Job drawing, mm, ordinate dimensions from the low corner. One solid piece. A direction names the side the tool comes from. Give positions to 0.01 mm unless a question says otherwise; leave off trailing zeros. Order: outer loops, then holes, each group sorted by start corner. A loop starts at its lowest first (then second) coordinate and runs counter-clockwise, first axis right, second up. Notation, with made-up numbers: M 59.5,48 L 78.5,48 A17 cw 78.5,52 Z; hole C -37.75,0 d5. An arc over 180 degrees is marked long. Use CSV: the item, a comma, the result in double quotes. Start each with the question number.
Item 1: Band-saw the part on D-D on y = 2. Write the cut outline in (x, z).
Item 2: Band-saw the part on B-B on z = 5. Write the cut outline in (x, y), plus the area to 3 significant figures.
Item 3: Which spindle directions (+Z, -Z, +X, -X, +Y, -Y) get a long thin tool onto all of the face, cutting with end or side? Do the marked faces 4, 5 and 6. Say none if no direction does.
Item 4: Wall check: line 1 along X through (y, z) = (17.6, 25) (1 decimal); line 2 along Y through (x, z) = (17.5, 43); line 3 along Z through (x, y) = (14.5, 15.75) (1 decimal). Give the ranges that are in metal, low to high.
Item 5: Two-plate mould, pull along X, no slides. Class the marked faces 1, 2 and 3: pulls with the +X half, pulls with the -X half, needs draft (parallel to the pull), parting line crosses it, or undercut.
Item 6: Pin check, flat tips, straight feed: P1, Ø6, axis at x = 33, y = 9.5, coming from the +Z side; P2, Ø3.5, axis at x = 24, y = 12.5, coming from the -Z side; P3, Ø3.5, axis at x = 5, z = 25, coming from the +Y side. Stop position of each tip, or through.
Item 7: Band-saw the part on A-A on x = 5. Write the cut outline in (y, z).
Item 8: Band-saw the part on C-C on x = 25. Write the cut outline in (y, z).
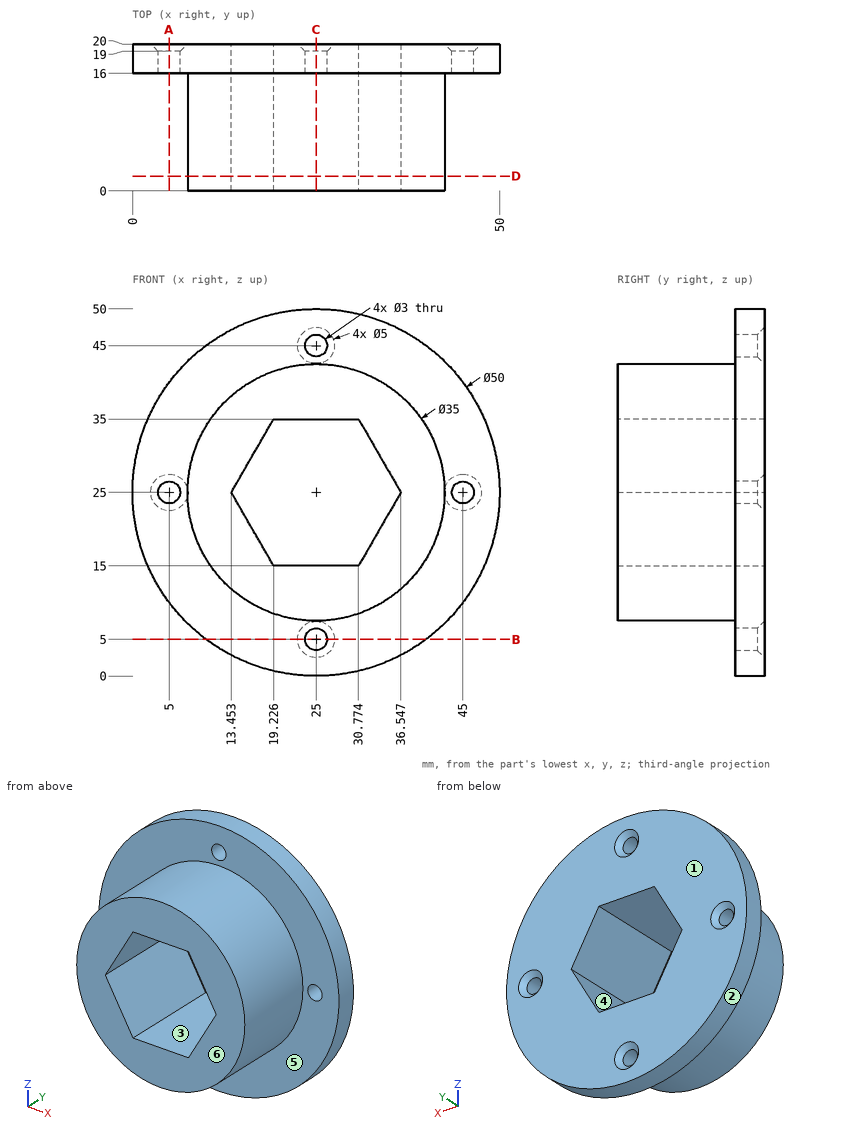
Model answer:
1,outline,"C 25,25 d35; hole M 13.45,25 L 19.23,15 L 30.77,15 L 36.55,25 L 30.77,35 L 19.23,35 Z"
2,outline,"M 10,16 L 23.5,16 L 23.5,19 L 22.5,20 L 10,20 Z; M 26.5,16 L 40,16 L 40,20 L 27.5,20 L 26.5,19 Z"
2,area,"107 mm^2"
3,face 4,"+Y, -Y"
3,face 5,"-Y"
3,face 6,"+Z, -Z, +X, -X, -Y"
4,line 1,"x = 0 to 3.5, 6.5 to 13.5, 36.5 to 43.5, 46.5 to 50"
4,line 2,"y = 16 to 20"
4,line 3,"z = 11 to 23.2, 26.8 to 39"
5,face 1,"needs draft"
5,face 2,"parting line crosses it"
5,face 3,"undercut"
6,P1,"stops at z = 41.77"
6,P2,"stops at z = 7.5"
6,P3,"stops at y = 19.25"
7,outline,"M 16,10 L 20,10 L 20,22.5 L 19,23.5 L 16,23.5 Z; M 16,26.5 L 19,26.5 L 20,27.5 L 20,40 L 16,40 Z"
8,outline,"M 0,7.5 L 16,7.5 L 16,6.5 L 19,6.5 L 20,7.5 L 20,15 L 0,15 Z; M 0,35 L 20,35 L 20,42.5 L 19,43.5 L 16,43.5 L 16,42.5 L 0,42.5 Z; M 16,0 L 20,0 L 20,2.5 L 19,3.5 L 16,3.5 Z; M 16,46.5 L 19,46.5 L 20,47.5 L 20,50 L 16,50 Z"
